```python
from build123d import *

# Parameters (mm, degrees)
SKETCH_1_W                       = 2
SKETCH_1_H                       = 75
SM_BASE_FLANGE_1_DEPTH           = 35
SM_EDGE_FLANGE_1_STRIP_W         = 9
SM_EDGE_FLANGE_1_STRIP_H         = 2
SM_EDGE_FLANGE_1_STRIP_CUT_DEPTH = 75
SM_EDGE_FLANGE_1_DEPTH           = 75
CUT_EXTRUDE_1_DEPTH              = 2
SM_EDGE_FLANGE_2_DEPTH           = 60
SM_EDGE_FLANGE_3_STRIP_W         = 9
SM_EDGE_FLANGE_3_STRIP_H         = 2
SM_EDGE_FLANGE_3_STRIP_CUT_DEPTH = 39.5
SM_EDGE_FLANGE_3_DEPTH           = 39.5
SM_EDGE_FLANGE_4_STRIP_W         = 9
SM_EDGE_FLANGE_4_STRIP_H         = 2
SM_EDGE_FLANGE_4_STRIP_CUT_DEPTH = 82
SM_EDGE_FLANGE_4_DEPTH           = 82
SM_EDGE_FLANGE_5_DEPTH           = 38
SKETCH_18_R                      = 4.35
EXTRUDE_1_DEPTH                  = 2
HOLE_WIZARD_M5_1_D               = 4.2
HOLE_WIZARD_M5_1_DEPTH           = 33.751449569
PATTERN_LINEAR_1_COUNT           = 2
PATTERN_LINEAR_1_PITCH           = 20
PATTERN_LINEAR_1_COUNT_DIR2      = 2
PATTERN_LINEAR_1_PITCH_DIR2      = 35
SKETCH_26_W                      = 34.5
SKETCH_26_H                      = 25
SM_BASE_FLANGE_1_2_DEPTH         = 2
CUT_EXTRUDE_2_DEPTH              = 2
CHAMFER_1_SIZE                   = 3


# Sheet-metal steps are written as plain solids
with BuildPart() as part:
    # Sketch 1 → Sm Base Flange 1 (new body)
    with BuildSketch(Plane.XY):
        with Locations((1, 0)):
            Rectangle(SKETCH_1_W, SKETCH_1_H)
    extrude(amount=SM_BASE_FLANGE_1_DEPTH)

    # 边线-法兰1 strip (across the edge) → 边线-法兰1 strip cut (cut)
    with BuildSketch(Plane(origin=(2, -37.5, 0), x_dir=(0, 0, 1), z_dir=(0, 1, 0))):
        with Locations((-4, -1)):
            Rectangle(SM_EDGE_FLANGE_1_STRIP_W, SM_EDGE_FLANGE_1_STRIP_H)
    extrude(amount=SM_EDGE_FLANGE_1_STRIP_CUT_DEPTH, mode=Mode.SUBTRACT)

    # 边线-法兰1 section (across the edge) → 边线-法兰1 (add)
    with BuildSketch(Plane(origin=(2, -37.5, 0), x_dir=(0, 0, 1), z_dir=(0, 1, 0))):
        with BuildLine():
            Line((-2, 0.5), (-2, 84))
            Line((-2, 84), (0, 84))
            Line((0, 84), (0, 0.5))
            ThreePointArc((0, 0.5), (0.146446609, 0.146446609), (0.5, 0))
            Line((0.5, 0), (0.5, -2))
            ThreePointArc((0.5, -2), (-1.267766953, -1.267766953), (-2, 0.5))
        make_face()
    extrude(amount=SM_EDGE_FLANGE_1_DEPTH)

    # 草图6 → 切除-拉伸1 (cut)
    with BuildSketch(Plane(origin=(0, 0, -2), x_dir=(-1, 0, 0), z_dir=(0, 0, -1))):
        Polygon((-84.5, 35.5), (-25, -24), (-25, -37.5), (-86, -37.5), (-86, 37.5), (-84.5, 37.5), align=None)
    extrude(amount=-CUT_EXTRUDE_1_DEPTH, mode=Mode.SUBTRACT)

    # 边线-法兰2 section (across the edge) → 边线-法兰2 (add)
    with BuildSketch(Plane(origin=(84.853553391, 35.146446609, -2), x_dir=(-0.7071067811865437, 0.7071067811865513, -1.0226318000689522e-15), z_dir=(-0.7071067811865513, -0.7071067811865437, 2.468731249046521e-15))):
        with BuildLine():
            Line((-2, 0.5), (-2, 40))
            Line((-2, 40), (0, 40))
            Line((0, 40), (0, 0.5))
            ThreePointArc((0, 0.5), (0.146446609, 0.146446609), (0.5, 0))
            Line((0.5, 0), (0.5, -2))
            ThreePointArc((0.5, -2), (-1.267766953, -1.267766953), (-2, 0.5))
        make_face()
    extrude(amount=SM_EDGE_FLANGE_2_DEPTH)

    # 边线-法兰3 strip (across the edge) → 边线-法兰3 strip cut (cut)
    with BuildSketch(Plane(origin=(84.853553391, 35.146446609, -2.5), x_dir=(-0.7071067811865538, -0.7071067811865412, 2.111674983989249e-15), z_dir=(0, 0, -1))):
        with Locations((-4, -1)):
            Rectangle(SM_EDGE_FLANGE_3_STRIP_W, SM_EDGE_FLANGE_3_STRIP_H)
    extrude(amount=SM_EDGE_FLANGE_3_STRIP_CUT_DEPTH, mode=Mode.SUBTRACT)

    # 边线-法兰3 section (across the edge) → 边线-法兰3 (add)
    with BuildSketch(Plane(origin=(84.853553391, 35.146446609, -2.5), x_dir=(-0.7071067811865538, -0.7071067811865412, 2.111674983989249e-15), z_dir=(0, 0, -1))):
        with BuildLine():
            Line((-2, 0.5), (-2, 10))
            Line((-2, 10), (0, 10))
            Line((0, 10), (0, 0.5))
            ThreePointArc((0, 0.5), (0.146446609, 0.146446609), (0.5, 0))
            Line((0.5, 0), (0.5, -2))
            ThreePointArc((0.5, -2), (-1.267766953, -1.267766953), (-2, 0.5))
        make_face()
    extrude(amount=SM_EDGE_FLANGE_3_DEPTH)

    # 边线-法兰4 strip (across the edge) → 边线-法兰4 strip cut (cut)
    with BuildSketch(Plane(origin=(84.5, 37.5, 0), x_dir=(0, -1, 0), z_dir=(-1, 0, 0))):
        with Locations((-4, -1)):
            Rectangle(SM_EDGE_FLANGE_4_STRIP_W, SM_EDGE_FLANGE_4_STRIP_H)
    extrude(amount=SM_EDGE_FLANGE_4_STRIP_CUT_DEPTH, mode=Mode.SUBTRACT)

    # 边线-法兰4 section (across the edge) → 边线-法兰4 (add)
    with BuildSketch(Plane(origin=(84.5, 37.5, 0), x_dir=(0, -1, 0), z_dir=(-1, 0, 0))):
        with BuildLine():
            Line((-2, 0.5), (-2, 10))
            Line((-2, 10), (0, 10))
            Line((0, 10), (0, 0.5))
            ThreePointArc((0, 0.5), (0.146446609, 0.146446609), (0.5, 0))
            Line((0.5, 0), (0.5, -2))
            ThreePointArc((0.5, -2), (-1.267766953, -1.267766953), (-2, 0.5))
        make_face()
    extrude(amount=SM_EDGE_FLANGE_4_DEPTH)

    # 边线-法兰5 section (across the edge) → 边线-法兰5 (add)
    with BuildSketch(Plane(origin=(42.073593129, -7.633513652, -42), x_dir=(0.7071067811865489, 0.7071067811865461, -2.23589115951803e-15), z_dir=(0, 0, 1))):
        with BuildLine():
            Line((-2, 0.5), (-2, 10))
            Line((-2, 10), (0, 10))
            Line((0, 10), (0, 0.5))
            ThreePointArc((0, 0.5), (0.146446609, 0.146446609), (0.5, 0))
            Line((0.5, 0), (0.5, -2))
            ThreePointArc((0.5, -2), (-1.267766953, -1.267766953), (-2, 0.5))
        make_face()
    extrude(amount=SM_EDGE_FLANGE_5_DEPTH)

    # 草图18 → 凸台-拉伸1 (add)
    with BuildSketch(Plane(origin=(24.853553391, -24.853553391, 0), x_dir=(0, 0, 1), z_dir=(-0.7071067811865436, 0.7071067811865515, -1.027306589177874e-15))):
        with Locations(Location((-33, 74.352813742, 0), (0, 0, 270))):
            Circle(SKETCH_18_R)
    extrude_1 = extrude(amount=EXTRUDE_1_DEPTH)

    # M5 螺纹孔1
    with Locations(Plane(origin=(23.439339828, -23.439339828, 0), x_dir=(-0.7071067811865515, -0.7071067811865436, 1.0273065891778625e-15), z_dir=(-0.7071067811865436, 0.7071067811865515, -1.027306589177874e-15))):
        with Locations((-74.352813742, -33)):
            hole_wizard_m5_1 = Hole(HOLE_WIZARD_M5_1_D / 2, depth=HOLE_WIZARD_M5_1_DEPTH)

    # 阵列(线性)1: 凸台-拉伸1, Hole Wizard M5 _1 2 × 2
    with Locations(*[Vector(0, 0, 1) * (i * PATTERN_LINEAR_1_PITCH) + Vector(-0.7071067811865475, -0.7071067811865477, 1.982541115402065e-15) * (j * PATTERN_LINEAR_1_PITCH_DIR2) for i in range(PATTERN_LINEAR_1_COUNT) for j in range(PATTERN_LINEAR_1_COUNT_DIR2) if (i, j) != (0, 0)]):
        add(extrude_1)
        add(hole_wizard_m5_1, mode=Mode.SUBTRACT)

    # 草图26 → Sm Base Flange 1 2 (add)
    with BuildSketch(Plane.ZY):
        with Locations((17.75, 50)):
            Rectangle(SKETCH_26_W, SKETCH_26_H)
    extrude(amount=-SM_BASE_FLANGE_1_2_DEPTH)

    # 草图16 → 切除-拉伸2 (cut)
    with BuildSketch(Plane.ZY):
        with BuildLine():
            Line((17, -22.25), (23, -22.25))
            ThreePointArc((23, -22.25), (26.25, -25.5), (23, -28.75))
            Line((23, -28.75), (17, -28.75))
            ThreePointArc((17, -28.75), (13.75, -25.5), (17, -22.25))
        make_face()
        with BuildLine():
            Line((17, 52.75), (23, 52.75))
            ThreePointArc((23, 52.75), (26.25, 49.5), (23, 46.25))
            Line((23, 46.25), (17, 46.25))
            ThreePointArc((17, 46.25), (13.75, 49.5), (17, 52.75))
        make_face()
    extrude(amount=-CUT_EXTRUDE_2_DEPTH, mode=Mode.SUBTRACT)

    # 倒角1
    chamfer_1_edges = [part.edges().sort_by_distance(p)[0] for p in [
        (78.48959236, 42.924621202, -2.5),
        (78.48959236, 42.924621202, -42),
        (84.5, 38.5, 10),
        (2.5, 38.5, 10),
        (34.295418536, -1.269552622, -42),
        (34.295418536, -1.269552622, -4),
        (1, 62.5, 35),
        (25, -37.5, -1),
        (1, -37.5, 35),
    ]]
    chamfer(chamfer_1_edges, length=CHAMFER_1_SIZE)


solid = part.part
```
Build history of the part. All positions in model axes, mm. A direction names the side the tool comes from. Give positions to 0.01 mm unless a question says otherwise; leave off trailing zeros. Loops run counter-clockwise (first coordinate to the right, second up) from the corner with the lowest first, then second, coordinate; pieces in that order, holes last.
Item 1: Slice it at B-B, the plane y = 49.5. List the corners of the cut face in (x, z), and give its area (3 significant figures).
Answers follow:
outline: (0, 0.5) - (2, 0.5) - (2, 13.75) - (0, 13.75) - close; (0, 26.25) - (2, 26.25) - (2, 35) - (0, 35) - close
area: 44.0 mm2
Item 2: Slice it at C-C, the plane y = -25.5. List the corners of the cut face in (x, z).
Answers follow:
outline: (0, 0.5) arc R2.5 ccw to (2.5, -2) - (25, -2) - (25, 0) - (2.5, 0) arc R0.5 cw to (2, 0.5) - (2, 13.75) - (0, 13.75) - close; (0, 26.25) - (2, 26.25) - (2, 35) - (0, 35) - close
Item 3: Flat gauge pins, fed straight in: pin 1 (2 mm diameter, centred on x = 1, z = -1, fed in from +Y); pin 2 (10 mm diameter, centred on y = 7.5, z = -5, fed in from -X); pin 3 (4 mm diameter, centred on x = 43, z = -28.5, fed in from +Y); pin 4 (1 mm diameter, centred on y = -14, z = -3, fed in from +X). Where does each tip first touch, or does it go through?
Answers follow:
pin 1: stops at y = 37.5
pin 2: stops at x = 0.05
pin 3: stops at y = -4.71
pin 4: passes through
Item 4: Slice it at A-A, the plane z = 20.5. List the corners of the cut face in (x, y).
Answers follow:
outline: (0, -37.5) - (2, -37.5) - (2, -28.75) - (0, -28.75) - close; (0, -22.25) - (2, -22.25) - (2, 46.25) - (0, 46.25) - close; (0, 52.75) - (2, 52.75) - (2, 62.5) - (0, 62.5) - close
Item 5: Drill centre lines: line 1 (X direction, y = 34, z = 12); line 2 (Z direction, x = 45.5, y = -4.5); line 3 (X direction, y = 35.5, z = -35.5). Where is each one in solid material? Low to high.
Answers follow:
line 1: x = 0 to 2
line 2: z = -42 to -0.1
line 3: x = 84.5 to 86.62
Item 6: Which spindle directions (+Z, -Z, +X, -X, +Y, -Y) get a long thin tool onto all of the face, cutting with end or side? Do faces 1 (the face through (63.758, 14.051, -22.526)), 2 (the face through (81, 39, -22)), 3 (the face through (36.99, -5.38, -23.27)), 4 (the face through (2, 37.5, 0)), 5 (the face through (0.99, -25.43, 26.25)). Say none if no direction does.
Answers follow:
face 1: none
face 2: -Z, -X
face 3: -Z, -X, -Y
face 4: -Z, -X, +Y
face 5: +X, -X
Item 7: Pull direction Z, two halves, no side cores. Call faces 6 (the face through (40, -7, -4)), 7 (the face through (38.31, -3.87, -23.27)), 8 (the face through (79.55, 41.89, -4.02)), 9 (the face through (73.798, 25.485, -11.693)): released by +Z, released by -Z, zero draft, split by the parting line, or undercut.
Answers follow:
face 6: undercut
face 7: zero draft
face 8: released by +Z
face 9: undercut
